Here's how the part is built. I have some questions about the finished solid (model axes, mm). Coordinates: 2 decimals unless noted, no trailing zeros. Order: outer loops, then holes, each group sorted by start corner. A loop starts at its lowest first (then second) coordinate and runs counter-clockwise, first axis right, second up. Notation, with made-up numbers: (-30.75, 33) - (-23.75, 33) arc R17 cw to (-23.75, 64) - close; hole circle Ø3 at (25, 72.5). An arc over 180 degrees is marked (long way). Answer as CSV lines item,"result". Start each with the question number.
Q1. Suppose I cut it at A-A (z = 1.1). Count the separate pieces of the cut face and the enclosed holes in it, then the cut area to 3 significant figures.
Q2. Thinking about a two-plate mould opening in Y: for faces 1 (the face through (0, 1, 3.175)), 2 (the face through (7.73, 75.09, 1.57)), which applies, released by +Y, released by -Y, zero draft, split by the parting line, or undercut?
Q3. For pin 1 Ø2.5 at (x, y) = (0, 83.4) entering from -Z; pin 2 Ø1.5 at (x, z) = (-7.5, 2) entering from -Y, each with a flat end and sliding along its axis, tell me the tip position at first contact or that it passes through.
Q4. Suppose I cut it at C-C (x = 10). Please give me the cut outline in (y, z) (3 decimals).
Q5. Suppose I cut it at D-D (x = -10.25). Please give me the cut outline in (y, z) (3 decimals).
Q6. I need wall thicknesses on line 1 (X direction, y = 76.4, z = 2.05); line 2 (Y direction, x = -0.25, z = 1.15); line 3 (Y direction, x = 8, z = 2.45). Which ranges of each line are inside material? Lowest first, please.
Q7. Suppose I cut it at B-B (y = -83.4). Please give me the cut outline in (x, z) (3 decimals), then the cut area to 3 significant figures.
from build123d import *

# Parameters (mm, degrees)
F0_R     = 1.4732
F1_DEPTH = 3.175


# Not quite as in the source:
# - a length typed as a fraction of an inch, garbled in the dataset ("3 / 203.2 mm" for 3/8 in), is restored


with BuildPart() as f1:
    # F0 (on Top) → F1 (new body)
    with BuildSketch(Plane.XY):
        with BuildLine():
            Line((12.5, -76.4), (12.5, 76.4))
            ThreePointArc((12.5, 76.4), (8.8388347648, 85.2388347648), (0, 88.9))
            ThreePointArc((0, 88.9), (-8.8388347648, 85.2388347648), (-12.5, 76.4))
            Line((-12.5, 76.4), (-12.5, -76.4))
            ThreePointArc((-12.5, -76.4), (-8.8388347648, -85.2388347648), (0, -88.9))
            ThreePointArc((0, -88.9), (8.8388347648, -85.2388347648), (12.5, -76.4))
        make_face()
        with Locations((-7.0527177304, -76.4)):
            Circle(F0_R, mode=Mode.SUBTRACT)
        with Locations((0, -83.4)):
            Circle(F0_R, mode=Mode.SUBTRACT)
        with Locations((0, -69.4)):
            Circle(F0_R, mode=Mode.SUBTRACT)
        with Locations((7.0527177304, -76.4)):
            Circle(F0_R, mode=Mode.SUBTRACT)
        with Locations((-7.0527177304, 76.4)):
            Circle(F0_R, mode=Mode.SUBTRACT)
        with Locations((0, 69.4)):
            Circle(F0_R, mode=Mode.SUBTRACT)
        with Locations((0, 83.4)):
            Circle(F0_R, mode=Mode.SUBTRACT)
        with Locations((7.0527177304, 76.4)):
            Circle(F0_R, mode=Mode.SUBTRACT)
    extrude(amount=F1_DEPTH)


solid = f1.part
Here are the results:
1,separate pieces,"1"
1,enclosed holes,"8"
1,area,"4,260 mm²"
2,face 1,"zero draft"
2,face 2,"undercut"
3,pin 1,"passes through"
3,pin 2,"stops at y = -86.92"
4,outline,"(-83.9, 0) - (83.9, 0) - (83.9, 3.175) - (-83.9, 3.175) - close"
5,outline,"(-83.555, 0) - (83.555, 0) - (83.555, 3.175) - (-83.555, 3.175) - close"
6,line 1,"x = -12.5 to -8.53, -5.58 to 5.58, 8.53 to 12.5"
6,line 2,"y = -88.9 to -84.85, -81.95 to -70.85, -67.95 to 67.95, 70.85 to 81.95, 84.85 to 88.9"
6,line 3,"y = -86 to -77.53, -75.27 to 75.27, 77.53 to 86"
7,outline,"(-10.356, 0) - (-1.473, 0) - (-1.473, 3.175) - (-10.356, 3.175) - close; (1.473, 0) - (10.356, 0) - (10.356, 3.175) - (1.473, 3.175) - close"
7,area,"56.4 mm²"
